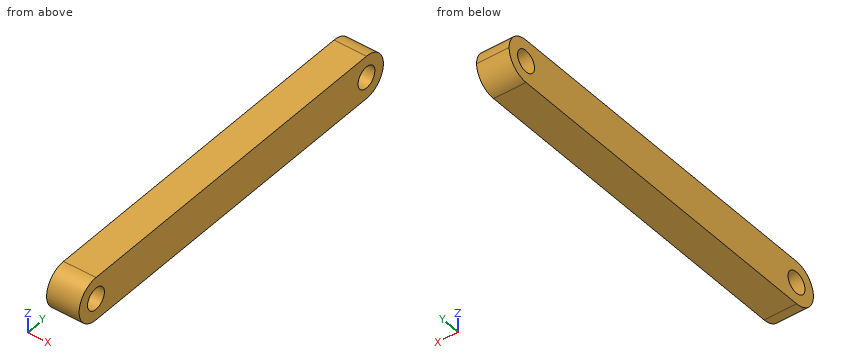
from build123d import *

# Parameters (mm, degrees)
F0_R     = 1.5875
F1_DEPTH = 4.7625


with BuildPart() as f1:
    # F0 (on Right) → F1 (new body)
    with BuildSketch(Plane.YZ):
        with BuildLine():
            ThreePointArc((0, 3.175), (2.245064, 2.245064), (3.175, 0))
            ThreePointArc((3.175, 0), (2.245064, -2.245064), (0, -3.175))
            Line((0, -3.175), (50.8, -3.175))
            ThreePointArc((50.8, -3.175), (47.625, 0), (50.8, 3.175))
            Line((50.8, 3.175), (0, 3.175))
        make_face()
        with BuildLine():
            ThreePointArc((0, -3.175), (2.245064, -2.245064), (3.175, 0))
            ThreePointArc((3.175, 0), (2.245064, 2.245064), (0, 3.175))
            ThreePointArc((0, 3.175), (-3.175, 0), (0, -3.175))
        make_face()
        Circle(F0_R, mode=Mode.SUBTRACT)
        with BuildLine():
            ThreePointArc((53.975, 0), (53.045064, 2.245064), (50.8, 3.175))
            ThreePointArc((50.8, 3.175), (47.625, 0), (50.8, -3.175))
            ThreePointArc((50.8, -3.175), (53.045064, -2.245064), (53.975, 0))
        make_face()
        with Locations((50.8, 0)):
            Circle(F0_R, mode=Mode.SUBTRACT)
    extrude(amount=F1_DEPTH)


solid = f1.part
Here's how the part is built. I have some questions about the finished solid (model axes, mm). Round coordinates to 2 decimals unless told otherwise and drop trailing zeros. Order: outer loops, then holes, each group sorted by start corner. A loop starts at its lowest first (then second) coordinate and runs counter-clockwise, first axis right, second up. Notation, with made-up numbers: M 5.5,16.5 L 30.5,16.5 A29 ccw 30.5,41.5 Z; hole C -12,-11 d1. An arc over 180 degrees is marked long. Return JSON: item names as keys, results as strings. Group by question number.
1. If we section it at B-B on z = -0.5: List the corners of the cut face in (x, y) for me.
2. If we section it at A-A on x = 1.4: State how many separate pieces and enclosed holes the cut face has, then the cut area to 3 significant figures.
3. I'm going to push flat-ended pins straight in: pin 1 Ø2 at (x, z) = (4, 2) entering from -Y; pin 2 Ø2 at (x, z) = (3, -2) entering from +Y. Where does each tip first touch, or does it pass through?
4. Please list where these lines run through material, in increasing order: probe 1 along Z at (x, y) = (3.55, 50.8) (1 decimal); probe 2 along Y at (x, z) = (4, -1.25); probe 3 along Z at (x, y) = (0.8, 50) (3 decimals).
Reply:
{
 "1": {"outline": "M 0,-3.14 L 4.76,-3.14 L 4.76,-1.51 L 0,-1.51 Z; M 0,1.51 L 4.76,1.51 L 4.76,49.29 L 0,49.29 Z; M 0,52.31 L 4.76,52.31 L 4.76,53.94 L 0,53.94 Z"},
 "2": {"separate pieces": "1", "enclosed holes": "2", "area": "338 mm^2"},
 "3": {"pin 1": "y = -3.01", "pin 2": "y = 53.81"},
 "4": {"probe 1": "-3.2 to -1.6, 1.6 to 3.2", "probe 2": "-2.92 to -0.98, 0.98 to 49.82, 51.78 to 53.72", "probe 3": "-3.175 to -1.371, 1.371 to 3.175"}
}
